Design review of the part built by this model. Coordinates are the model's own, in mm. Face numbers are marked on the shaded views. Give positions to 0.01 mm unless a question says otherwise; leave off trailing zeros. Loops run counter-clockwise (first coordinate to the right, second up) from the corner with the lowest first, then second, coordinate; pieces in that order, holes last. Notation, with made-up numbers: (62.25, 20.25) -> (77.25, 20.25) arc R22 ccw to (77.25, 57.25) -> close; hole circle Ø3 at (46.5, 1). An arc over 180 degrees is marked (long way). Use a Markdown table: item, result. Add a question column.
1. For pin 1 Ø3 at (x, y) = (0, 59.5) entering from +Z, flat-tipped, find the tip position at first contact; note if it passes through.
2. Add section C-C (z = 0). State the section outline as (x, y) points, and give its area (3 significant figures).
3. To check wall thickness, follow line 1 (Y direction, x = -17.5, z = 24); line 2 (Y direction, x = 5, z = -8); line 3 (Z direction, x = -0.5, y = 61). State the ranges of each line that lie inside material, in increasing order.
4. Add section B-B (x = 0). State the section outline as (y, z) points.
5. Draft analysis for pull direction Y (two halves, no side actions). For the marked faces 1, 2 and 3, state which applies: pulls with the +Y half, pulls with the -Y half, needs draft (parallel to the pull), parting line crosses it, or undercut.
6. Add section D-D (x = -13). State the section outline as (y, z) points.
7. Add section A-A (z = -14.5). State the section outline as (x, y) points, and give its area (3 significant figures).
```python
from build123d import *

# Parameters (mm, degrees)
SKETCH1_R           = 32.5
BOSS_EXTRUDE1_DEPTH = 5
SKETCH2_R           = 10
BOSS_EXTRUDE2_DEPTH = 2.5
SKETCH3_R           = 2.4
BOSS_EXTRUDE3_DEPTH = 95


with BuildPart() as part:
    # Sketch1 → Boss-Extrude1 (new, symmetric)
    with BuildSketch(Plane(origin=(0, 0, 0), x_dir=(1, 0, 0), z_dir=(0, 1, 0))):
        with Locations(Location((0, 0, 0), (0, 0, 270))):
            Circle(SKETCH1_R)
    extrude(amount=BOSS_EXTRUDE1_DEPTH, both=True)

    # Sketch2 → Boss-Extrude2 (add, symmetric)
    with BuildSketch(Plane(origin=(0, 5, 0), x_dir=(1, 0, 0), z_dir=(0, 1, 0))):
        with Locations(Location((0, 0, 0), (0, 0, 270))):
            Circle(SKETCH2_R)
    extrude(amount=BOSS_EXTRUDE2_DEPTH, both=True)

    # Sketch3 → Boss-Extrude3 (add)
    with BuildSketch(Plane(origin=(0, 7.5, 0), x_dir=(1, 0, 0), z_dir=(0, 1, 0))):
        with Locations(Location((0, 0, 0), (0, 0, 270))):
            Circle(SKETCH3_R)
    extrude(amount=BOSS_EXTRUDE3_DEPTH)

    # Mirror7: part across plane


with BuildPart() as part_1:
    add(part.part)
    add(part.part.mirror(Plane.ZX.offset(102.5)))


solid = part_1.part
```
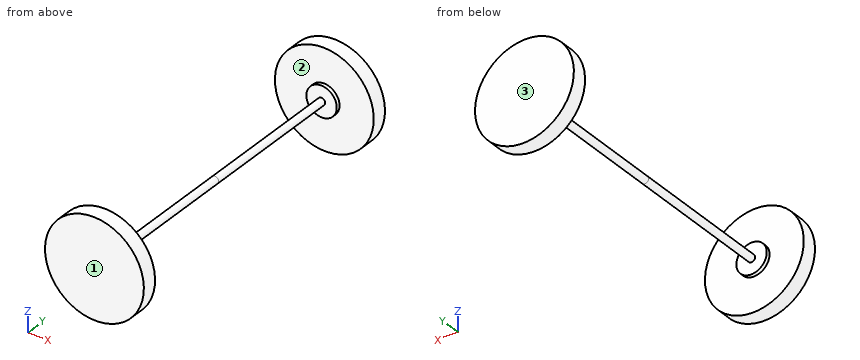
Taken from the geometry:
| question | item | result |
|---|---|---|
| 1 | pin 1 | stops at z = 2.4 |
| 2 | outline | (-32.5, -5) -> (32.5, -5) -> (32.5, 5) -> (10, 5) -> (10, 7.5) -> (2.4, 7.5) -> (2.4, 197.5) -> (10, 197.5) -> (10, 200) -> (32.5, 200) -> (32.5, 210) -> (-32.5, 210) -> (-32.5, 200) -> (-10, 200) -> (-10, 197.5) -> (-2.4, 197.5) -> (-2.4, 7.5) -> (-10, 7.5) -> (-10, 5) -> (-32.5, 5) -> close |
| 2 | area | 2,310 mm^2 |
| 3 | line 1 | y = -5 to 5, 200 to 210 |
| 3 | line 2 | y = -5 to 7.5, 197.5 to 210 |
| 3 | line 3 | z = -2.35 to 2.35 |
| 4 | outline | (-5, -32.5) -> (5, -32.5) -> (5, -10) -> (7.5, -10) -> (7.5, -2.4) -> (197.5, -2.4) -> (197.5, -10) -> (200, -10) -> (200, -32.5) -> (210, -32.5) -> (210, 32.5) -> (200, 32.5) -> (200, 10) -> (197.5, 10) -> (197.5, 2.4) -> (7.5, 2.4) -> (7.5, 10) -> (5, 10) -> (5, 32.5) -> (-5, 32.5) -> close |
| 5 | face 1 | pulls with the -Y half |
| 5 | face 2 | undercut |
| 5 | face 3 | pulls with the +Y half |
| 6 | outline | (-5, -29.79) -> (5, -29.79) -> (5, 29.79) -> (-5, 29.79) -> close; (200, -29.79) -> (210, -29.79) -> (210, 29.79) -> (200, 29.79) -> close |
| 7 | outline | (-29.09, -5) -> (29.09, -5) -> (29.09, 5) -> (-29.09, 5) -> close; (-29.09, 200) -> (29.09, 200) -> (29.09, 210) -> (-29.09, 210) -> close |
| 7 | area | 1,160 mm^2 |
